from build123d import *

# Parameters (mm, degrees)
CUT_EXTRUDE1_DEPTH      = 44.520110294
CUT_EXTRUDE1_DEPTH_BACK = 44.520110294
SKETCH2_W               = 21.666012185
SKETCH2_H               = 9.766463862
CUT_EXTRUDE2_DEPTH      = 44.520110294
CUT_EXTRUDE2_DEPTH_BACK = 44.520110294
SKETCH3_R               = 1.5
CUT_EXTRUDE3_DEPTH      = 44.520110381
CUT_EXTRUDE3_DEPTH_BACK = 44.520110381
SKETCH4_W               = 24.279573728
SKETCH4_H               = 56.824995672


with BuildPart() as part:
    # Sketch1 → Revolve1 (revolve)
    with BuildSketch(Plane.XY, mode=Mode.PRIVATE) as revolve1_sk:
        Polygon((0, 0), (0, 38), (5, 38), (5, 13), (15, 13), (15, 9), (7.5, 9), (7.5, 4), (12.5, 4), (12.5, 0), align=None)
    revolve(revolve1_sk.sketch.rotate(Axis((0, 0, 0), (0, 1, 0)), 90), axis=Axis((0, 0, 0), (0, 1, 0)))

    # Sketch2 → Cut-Extrude1 (cut, two sides: drawn at the far end of the back side and taken through both)
    with BuildSketch(Plane.XY.offset(-CUT_EXTRUDE1_DEPTH_BACK)):
        with Locations((15.833006093, -0.883231931)):
            Rectangle(SKETCH2_W, SKETCH2_H)
    extrude(amount=CUT_EXTRUDE1_DEPTH + CUT_EXTRUDE1_DEPTH_BACK, mode=Mode.SUBTRACT)

    # Sketch3 → Cut-Extrude2 (cut, two sides: drawn at the far end of the back side and taken through both)
    with BuildSketch(Plane(origin=(0, 0, 0), x_dir=(0, 0, -1), z_dir=(1, 0, 0)).offset(-CUT_EXTRUDE2_DEPTH_BACK)):
        with Locations((0, 30)):
            Circle(SKETCH3_R)
    extrude(amount=CUT_EXTRUDE2_DEPTH + CUT_EXTRUDE2_DEPTH_BACK, mode=Mode.SUBTRACT)

    # Sketch4 → Cut-Extrude3 (cut, two sides: drawn at the far end of the back side and taken through both)
    with BuildSketch(Plane.XY.offset(-CUT_EXTRUDE3_DEPTH_BACK)):
        with Locations((-12.139786864, 22.787379867)):
            Rectangle(SKETCH4_W, SKETCH4_H)
    extrude(amount=CUT_EXTRUDE3_DEPTH + CUT_EXTRUDE3_DEPTH_BACK, mode=Mode.SUBTRACT)


solid = part.part
Can you work these out from the model? Positions are in its coordinate system, mm. A direction names the side the tool comes from. Coordinates: 2 decimals unless noted, no trailing zeros. Write each loop counter-clockwise with the first axis right and the second up, starting at its lowest first coordinate (ties: lowest second). Pieces come first, ordered by that corner, then holes. Notation, with made-up numbers: (-7, 14) -> (8, 14) arc R24 ccw to (8, 44) -> close; hole circle Ø7 at (-19, -4.75). An arc over 180 degrees is marked (long way). Answer as CSV lines item,"result".
1) On a 3-axis mill with a long thin cutter (end or side, diameter ignored), from which of +Z, -Z, +X, -X, +Y, -Y can I reach the whole of each face in a straight line? I mean faces 1 (the cylindrical face through (5, 25, 0)), 2 (the flat face through (9, 9, 0)), 3 (the flat face through (2, 4, 10)), 4 (the flat face through (5, 2, 0)), 5 (the cylindrical face through (2.59, 1.97, -12.23)). Say none if no direction works.
Check result:
face 1,"+X, +Y"
face 2,"+X"
face 3,"+Z, +X"
face 4,"+Z, -Z, +X, -Y"
face 5,"-Z, +X, -Y"
2) If we section it at C-C on z = -6.5: Please give me the cut outline in (x, y), then the cut area to 3 significant figures.
Check result:
outline,"(0, 0) -> (5, 0) -> (5, 4) -> (3.74, 4) -> (3.74, 9) -> (13.52, 9) -> (13.52, 13) -> (0, 13) -> close"
area,"92.8 mm²"
3) If I drill on line 1 (Y direction, x = 2.15, z = 0); line 2 (Y direction, x = 3.5, z = 8.25); line 3 (Y direction, x = 11, z = 8.5), over which ranges is the centre line in solid material (lowest first)? Write a range as from..to.
Check result:
line 1,"0..28.5, 31.5..38"
line 2,"0..4, 9..13"
line 3,"9..13"
4) If we section it at D-D on y = 11: Please give me the cut outline in (x, z).
Check result:
outline,"(0, -15) arc R15 ccw to (0, 15) -> close"
5) If we mould it in two halves opening along Y, with no side actions, what happens to faces 6 (the cylindrical face through (2.519, 1.972, 12.244)), 7 (the flat face through (7, 13, 0)), 8 (the cylindrical face through (7.5, 6.46, 0.16)), 9 (the flat face through (6, 4, 0))? For each: +Y half, -Y half, draft (parallel to the pull), parting line (faces both ways), or undercut.
Check result:
face 6,"draft"
face 7,"+Y half"
face 8,"undercut"
face 9,"-Y half"
6) If we section it at A-A on z = 0: Please give me the cut outline in (x, y).
Check result:
outline,"(0, 0) -> (5, 0) -> (5, 4) -> (7.5, 4) -> (7.5, 9) -> (15, 9) -> (15, 13) -> (5, 13) -> (5, 28.5) -> (0, 28.5) -> close; (0, 31.5) -> (5, 31.5) -> (5, 38) -> (0, 38) -> close"
7) If we section it at B-B on y = 30: Please give me the cut outline in (x, z), then the cut area to 3 significant figures.
Check result:
outline,"(0, -5) arc R5 ccw to (4.77, -1.5) -> (0, -1.5) -> close; (0, 1.5) -> (4.77, 1.5) arc R5 ccw to (0, 5) -> close"
area,"24.5 mm²"
8) Will these pins go through, and if not, where does the flat tip stop? P1, Ø8, axis at x = 9.5, y = 22, coming from the -Z side; P2, Ø0.7, axis at x = 6, z = -0.5, coming from the -Y side; P3, Ø8, axis at x = 8, z = 7.5, coming from the +Y side; P4, Ø1.2, axis at y = 2, z = -3, coming from the +X side.
Check result:
P1,"through"
P2,"y = 4"
P3,"y = 13"
P4,"x = 5"
